Source: three-view drawing plus pictorial views. Frame: mm from the lowest corner of the part. Give positions to 0.01 mm unless a question says otherwise; leave off trailing zeros. Loops run counter-clockwise (first coordinate to the right, second up) from the corner with the lowest first, then second, coordinate; pieces in that order, holes last. Notation, with made-up numbers: (80.25, -10.75) -> (86.25, -10.75) arc R7 ccw to (86.25, -5.75) -> close; hole circle Ø3 at (71.25, 69.25). An arc over 180 degrees is marked (long way). Put each result on its own line as item: value.
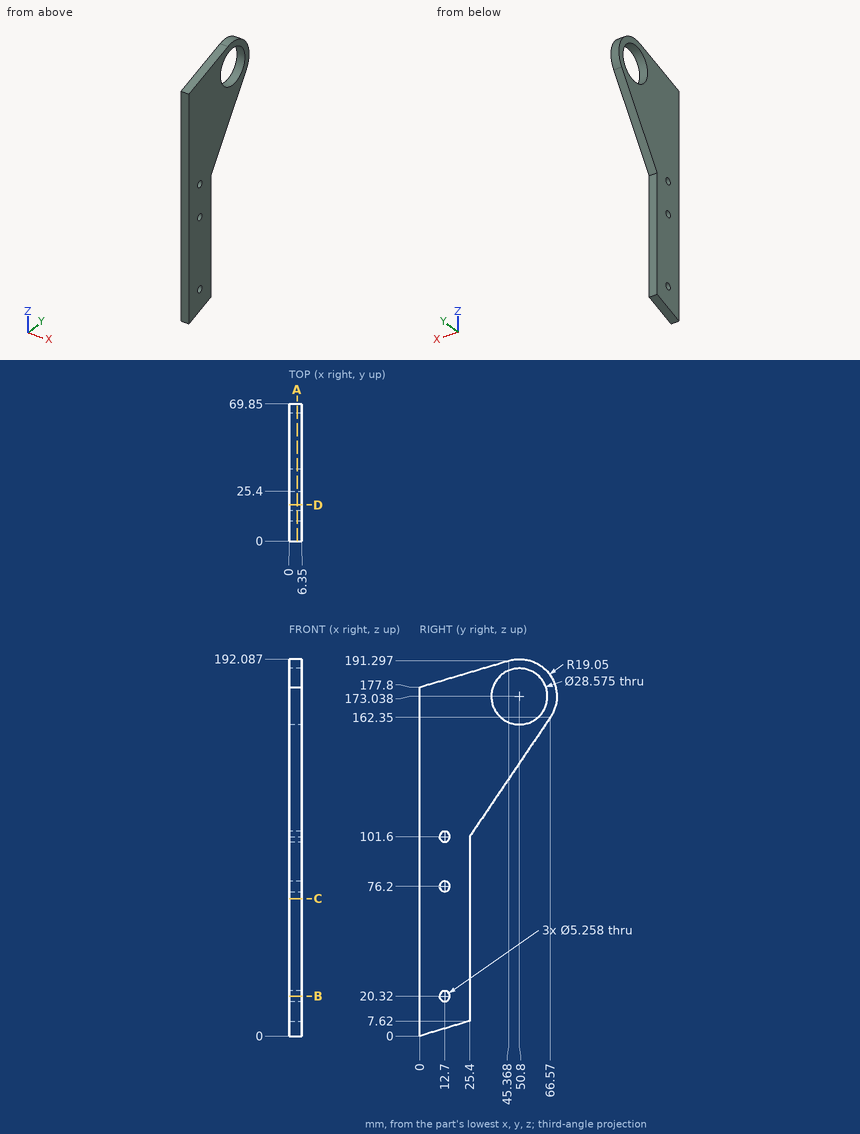
(1) First-contact query: P1, Ø1.9, axis at x = 2, z = 78, coming from the +Y side; P2, Ø1.5, axis at x = 0.5, z = 169.5, coming from the +Y side (1 decimal); P3, Ø12, axis at y = 37, z = 139.5, coming from the -X side; P4, Ø1.5, axis at x = 5.5, z = 120, coming from the +Y side. Flat tips, straight axial feed; report the tip coordinate or a pass-through.
Calculated:
P1: stops at y = 25.4
P2: stops at y = 69.6
P3: stops at x = 0
P4: stops at y = 38.38
(2) Section B-B on z = 20.32. Return loops of the section in (x, y).
Calculated:
outline: (0, 0) -> (6.35, 0) -> (6.35, 10.07) -> (0, 10.07) -> close; (0, 15.33) -> (6.35, 15.33) -> (6.35, 25.4) -> (0, 25.4) -> close
(3) Section A-A on x = 4. Give the number of separate pieces and of enclosed holes in the cut face.
Calculated:
separate pieces: 1
enclosed holes: 4
(4) Section C-C on z = 70. Return loops of the section in (x, y), then the cut area to 3 significant figures.
Calculated:
outline: (0, 0) -> (6.35, 0) -> (6.35, 25.4) -> (0, 25.4) -> close
area: 161 mm²
(5) Section D-D on y = 18.5. Return loops of the section in (x, z).
Calculated:
outline: (0, 5.55) -> (6.35, 5.55) -> (6.35, 183.3) -> (0, 183.3) -> close
(6) Line query: probe 1 along Y at (x, z) = (3.25, 76.2); probe 2 along Y at (x, z) = (5.5, 8.5); probe 3 along Z at (x, y) = (2, 49.5) (1 decimal). Output: solid intervals per line, ascending. Write a range as from..to.
Calculated:
probe 1: y = 0..10.07, 15.33..25.4
probe 2: y = 0..25.4
probe 3: z = 137.2..158.8, 187.3..192
